from build123d import *

# Parameters (mm, degrees)
SKETCH1_W           = 33
SKETCH1_H           = 31.5
SKETCH1_R           = 5
SKETCH1_R_2         = 1.65
BOSS_EXTRUDE1_DEPTH = 3
SKETCH2_W           = 3
SKETCH2_H           = 31.5
BOSS_EXTRUDE2_DEPTH = 30
SKETCH3_R           = 1.5
SKETCH3_R_2         = 4
CUT_EXTRUDE1_DEPTH  = 30
FILLET3_R           = 15.75
FILLET4_R           = 3


with BuildPart() as part:
    # Sketch1 → Boss-Extrude1 (new body)
    with BuildSketch(Plane(origin=(0, 0, 0), x_dir=(1, 0, 0), z_dir=(0, 1, 0))):
        with Locations((16.5, 15.75)):
            Rectangle(SKETCH1_W, SKETCH1_H)
        with Locations(Location((18, 15.75, 0), (0, 0, 270))):
            Circle(SKETCH1_R, mode=Mode.SUBTRACT)
        with Locations(Location((25.05, 23.75, 0), (0, 0, 270))):
            Circle(SKETCH1_R_2, mode=Mode.SUBTRACT)
        with Locations(Location((10.95, 23.75, 0), (0, 0, 270))):
            Circle(SKETCH1_R_2, mode=Mode.SUBTRACT)
        with Locations(Location((25.05, 7.75, 0), (0, 0, 90))):
            Circle(SKETCH1_R_2, mode=Mode.SUBTRACT)
        with Locations(Location((10.95, 7.75, 0), (0, 0, 90))):
            Circle(SKETCH1_R_2, mode=Mode.SUBTRACT)
    extrude(amount=BOSS_EXTRUDE1_DEPTH)

    # Sketch2 → Boss-Extrude2 (add)
    with BuildSketch(Plane.XZ):
        with Locations((1.5, -15.75)):
            Rectangle(SKETCH2_W, SKETCH2_H)
    extrude(amount=BOSS_EXTRUDE2_DEPTH)

    # Sketch3 → Cut-Extrude1 (cut)
    with BuildSketch(Plane.ZY):
        with Locations((-24.25, -17)):
            Circle(SKETCH3_R)
        with Locations((-7.25, -17)):
            Circle(SKETCH3_R)
        with Locations((-15.75, -17)):
            Circle(SKETCH3_R_2)
    extrude(amount=-CUT_EXTRUDE1_DEPTH, mode=Mode.SUBTRACT)

    # Fillet3
    fillet3_edges = [part.edges().sort_by_distance(p)[0] for p in [
        (1.5, -30, 0),
        (1.5, -30, -31.5),
    ]]
    fillet(fillet3_edges, radius=FILLET3_R - 0.0001)  # a hair under: the kernel refuses the full size

    # Fillet4
    fillet4_edges = [part.edges().sort_by_distance(p)[0] for p in [
        (0, 3, -15.75),
    ]]
    fillet(fillet4_edges, radius=FILLET4_R)


solid = part.part
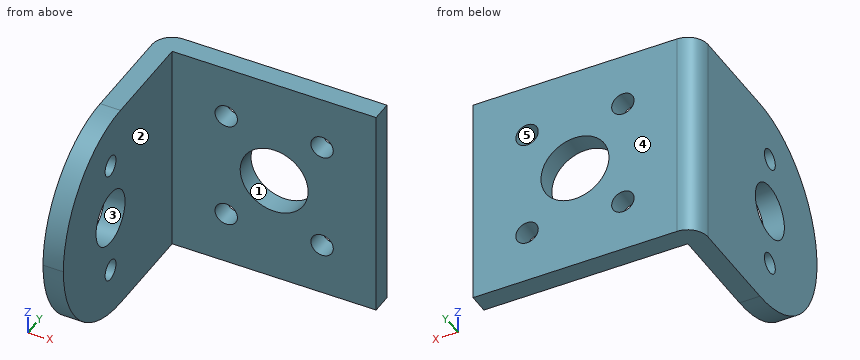
Geometry: final body of the model. Coordinates: model frame, mm. Face numbers are marked on the shaded views. A direction names the side the tool comes from. Round coordinates to 2 decimals unless told otherwise and drop trailing zeros. Loops run counter-clockwise (first coordinate to the right, second up) from the corner with the lowest first, then second, coordinate; pieces in that order, holes last.
Q1. Material intervals for L1, parallel to Z at x = 25, y = 2; L2, parallel to X at y = -19, z = -3, sorted ascending.
Q2. Section C-C on y = -19. Return loops of the section in (x, z), plus the area to 3 significant figures.
Q3. Access query for the marked faces 1 and 2. Directions: +Z, -Z, +X, -X, +Y, -Y. A direction counts if a zero-diameter tool reaches every point of the face in a straight line with its end or side. Return the directions, or none.
Q4. Section A-A on x = 18. Return loops of the section in (y, z), plus the area to 3 significant figures.
Q5. Section D-D on x = 11.5. Return loops of the section in (y, z).
Q6. Section B-B on z = -7.75. Return loops of the section in (x, y), plus the area to 3 significant figures.
Q7. Pull-direction query (Y, two-part tool) for the marked faces 3, 4 and 5; classes: released by +Y, released by -Y, zero draft, split by the parting line, or undercut.
Q8. Pin query (flat end, axial travel): P1, Ø5.5, axis at x = 10.95, z = -7.75, coming from the -Y side; P2, Ø10.5, axis at y = -17, z = -15.75, coming from the +X side. Return the tip coordinate at first contact, or that it passes through.
Evaluation:
1. L1: z = -31.5 to -25.4, -22.1 to -9.4, -6.1 to 0
1. L2: x = 0 to 3
2. outline: (0, -30.77) - (3, -30.77) - (3, -19.21) - (0, -19.21) - close; (0, -12.29) - (3, -12.29) - (3, -0.73) - (0, -0.73) - close
2. area: 69.3 mm2
3. face 1: +Y, -Y
3. face 2: +Z, -Z, +X, -Y
4. outline: (0, -31.5) - (3, -31.5) - (3, -20.75) - (0, -20.75) - close; (0, -10.75) - (3, -10.75) - (3, 0) - (0, 0) - close
4. area: 64.5 mm2
5. outline: (0, -31.5) - (3, -31.5) - (3, -25.31) - (0, -25.31) - close; (0, -22.19) - (3, -22.19) - (3, -9.31) - (0, -9.31) - close; (0, -6.19) - (3, -6.19) - (3, 0) - (0, 0) - close
6. outline: (0, -27.82) - (3, -27.82) - (3, -18.41) - (0, -18.41) - close; (0, -15.59) - (3, -15.59) - (3, 0) - (9.3, 0) - (9.3, 3) - (3, 3) arc R3 ccw to (0, 0) - close; (12.6, 0) - (23.4, 0) - (23.4, 3) - (12.6, 3) - close; (26.7, 0) - (33, 0) - (33, 3) - (26.7, 3) - close
6. area: 152 mm2
7. face 3: undercut
7. face 4: released by +Y
7. face 5: zero draft
8. P1: stops at y = 0
8. P2: stops at x = 3
